```python
from build123d import *

# Parameters (mm, degrees)
SKETCH_1_W          = 600
SKETCH_1_H          = 900
EXTRUDE_1_DEPTH     = 1.5
SKETCH_2_W          = 600
SKETCH_2_H          = 900
SKETCH_2_W_2        = 597
SKETCH_2_H_2        = 897
EXTRUDE_2_DEPTH     = 18.5
SKETCH_4_R          = 3.5
CUT_EXTRUDE_1_DEPTH = 10


with BuildPart() as part:
    # 草图1 → 凸台-拉伸1 (new body)
    with BuildSketch(Plane.XY):
        Rectangle(SKETCH_1_W, SKETCH_1_H)
    extrude(amount=EXTRUDE_1_DEPTH)

    # 草图2 → 凸台-拉伸2 (add)
    with BuildSketch(Plane(origin=(0, 0, 0), x_dir=(-1, 0, 0), z_dir=(0, 0, -1))):
        Rectangle(SKETCH_2_W, SKETCH_2_H)
        Rectangle(SKETCH_2_W_2, SKETCH_2_H_2, mode=Mode.SUBTRACT)
    extrude(amount=EXTRUDE_2_DEPTH)

    # 草图4 → 切除-拉伸1 (cut)
    with BuildSketch(Plane.XY.offset(1.5)):
        with Locations((-275, 425)):
            Circle(SKETCH_4_R)
        with Locations((275, 425)):
            Circle(SKETCH_4_R)
        with Locations((-275, -425)):
            Circle(SKETCH_4_R)
        with Locations((275, -425)):
            Circle(SKETCH_4_R)
    extrude(amount=-CUT_EXTRUDE_1_DEPTH, mode=Mode.SUBTRACT)


solid = part.part
```
Part model, mm, in its own coordinate system. A direction names the side the tool comes from. Give positions to 0.01 mm unless a question says otherwise; leave off trailing zeros. Order: outer loops, then holes, each group sorted by start corner. A loop starts at its lowest first (then second) coordinate and runs counter-clockwise, first axis right, second up. Notation, with made-up numbers: M 50.25,18 L 56.25,18 A9 ccw 56.25,24 Z; hole C 89.5,-2 d2. An arc over 180 degrees is marked long. Use a Markdown table: item, result. Add a question column.
(1) Saw through at C-C, the plane y = 117. Give the cut face in (x, z), and give its area (4 significant figures).
(2) Mould opens along X. For faces 3 (the face through (300, -6, -8)), 4 (the face through (4, -448.5, -9)), 5 (the face through (-4, 6, 1.5)) say: +X half, -X half, draft (parallel to the pull), parting line (faces both ways), or undercut.
(3) 3-axis set-ups, long thin cutter, end or side, ignore diameter. For faces 1 (the face through (-298.5, -6, -9)), 2 (the face through (-300, -6, -8)): which of +Z, -Z, +X, -X, +Y, -Y reach the whole face in a straight line?
(4) Saw through at A-A, the plane z = -7. Give the cut face in (x, y).
(5) Probe line 1 along X through (y, z) = (425, 0.7); line 2 along Y through (x, z) = (-275, 0.9); line 3 along Y through (x, z) = (33, -2). List the from-to ranges inside material, lowest first. Write a range as [from, to].
(6) Drop flat-ended pins along their axis: P1, Ø11, axis at x = 275, y = 425, coming from the -Z side; P2, Ø5.5, axis at x = -275, y = 425, coming from the -Z side. Give the stop position or say it passes through.
(7) Saw through at B-B, the plane x = 185. Give the cut face in (y, z).
Answer key:
| question | item | result |
|---|---|---|
| 1 | outline | M -300,-18.5 L -298.5,-18.5 L -298.5,0 L 298.5,0 L 298.5,-18.5 L 300,-18.5 L 300,1.5 L -300,1.5 Z |
| 1 | area | 955.5 mm^2 |
| 2 | face 3 | +X half |
| 2 | face 4 | undercut |
| 2 | face 5 | draft |
| 3 | face 1 | -Z |
| 3 | face 2 | +Z, -Z, -X, +Y, -Y |
| 4 | outline | M -300,-450 L 300,-450 L 300,450 L -300,450 Z; hole M -298.5,-448.5 L 298.5,-448.5 L 298.5,448.5 L -298.5,448.5 Z |
| 5 | line 1 | [-300, -278.5], [-271.5, 271.5], [278.5, 300] |
| 5 | line 2 | [-450, -428.5], [-421.5, 421.5], [428.5, 450] |
| 5 | line 3 | [-450, -448.5], [448.5, 450] |
| 6 | P1 | z = 0 |
| 6 | P2 | through |
| 7 | outline | M -450,-18.5 L -448.5,-18.5 L -448.5,0 L 448.5,0 L 448.5,-18.5 L 450,-18.5 L 450,1.5 L -450,1.5 Z |
